```python
from build123d import *

# Parameters (mm, degrees)
F0_R     = 7
F0_R_2   = 25
F1_DEPTH = 6
F2_R     = 10


with BuildPart() as f1:
    # F0 (on Top) → F1 (new body)
    with BuildSketch(Plane.XY):
        Polygon((-28.867513, 50), (-28.867513, -50), (57.735027, 0), align=None)
        with Locations((-18, -31.176915)):
            Circle(F0_R, mode=Mode.SUBTRACT)
        Circle(F0_R_2, mode=Mode.SUBTRACT)
        with Locations((-18, 31.176915)):
            Circle(F0_R, mode=Mode.SUBTRACT)
        with Locations((36, 0)):
            Circle(F0_R, mode=Mode.SUBTRACT)
    extrude(amount=F1_DEPTH)

    # F2
    f2_edges = [f1.edges().sort_by_distance(p)[0] for p in [
        (-28.867513, -50, 3),
        (57.735027, 0, 3),
        (-28.867513, 50, 3),
    ]]
    fillet(f2_edges, radius=F2_R)


solid = f1.part
```
The listing builds one solid part. Answer for the finished solid, in the listing's coordinates (mm). Round coordinates to 2 decimals unless told otherwise and drop trailing zeros. Loops run counter-clockwise (first coordinate to the right, second up) from the corner with the lowest first, then second, coordinate; pieces in that order, holes last. Notation, with made-up numbers: (-2.5, 12) - (9.5, 12) arc R20 ccw to (9.5, 28) - close; hole circle Ø2 at (3.25, 52.25). An arc over 180 degrees is marked (long way). Return JSON: item names as keys, results as strings. Group by question number.
1. The part is cut by section C-C on y = -26. Determine the outline of the cut face in (x, z), then the cut area to 3 significant figures.
2. The part is cut by section A-A on y = 0. Determine the outline of the cut face in (x, z), then the cut area to 3 significant figures.
3. Each of these flat-tipped pins is pushed along its axis until it touches: P1, Ø1.5, axis at x = 2.5, z = 4.5, coming from the -Y side; P2, Ø1, axis at y = -33.5, z = 2.5, coming from the -X side; P3, Ø1.5, axis at x = -9, z = 3.5, coming from the -Y side. Where does it stop, or does it pass through?
4. The part is cut by section B-B on x = -23. Determine the outline of the cut face in (y, z).
5. Consider probe 1 along Y at (x, z) = (-17, 5.1); probe 2 along Y at (x, z) = (-18, 2.95); probe 3 along Y at (x, z) = (32, 5.1). Determine where each line is inside the solid, lowest interval first.
6. The part is cut by section D-D on z = 1.05. Determine the outline of the cut face in (x, y), then the cut area to 3 significant figures.
7. The mould has two halves that part along Y. Classify faces 1 (the cylindrical face through (-24.993, -30.869, 2.958)), 2 (the flat face through (-16.3, 19.2, 6)), 3 (the flat face through (14.038, -25.229, 2.958)), 4 (the cylindrical face through (47.734, 0.147, 3.042)): pulls with the +Y half, pulls with the -Y half, needs draft (parallel to the pull), parting line crosses it, or undercut.
Resolved:
{
 "1": {"outline": "(-28.87, 0) - (-22.71, 0) - (-22.71, 6) - (-28.87, 6) - close; (-13.29, 0) - (12.7, 0) - (12.7, 6) - (-13.29, 6) - close", "area": "193 mm²"},
 "2": {"outline": "(-28.87, 0) - (-25, 0) - (-25, 6) - (-28.87, 6) - close; (25, 0) - (29, 0) - (29, 6) - (25, 6) - close; (43, 0) - (47.74, 0) - (47.74, 6) - (43, 6) - close", "area": "75.6 mm²"},
 "3": {"P1": "stops at y = -32.32", "P2": "stops at x = -28.86", "P3": "stops at y = -38.96"},
 "4": {"outline": "(-41.79, 0) - (-36.08, 0) - (-36.08, 6) - (-41.79, 6) - close; (-26.28, 0) - (-9.8, 0) - (-9.8, 6) - (-26.28, 6) - close; (9.8, 0) - (26.28, 0) - (26.28, 6) - (9.8, 6) - close; (36.08, 0) - (41.79, 0) - (41.79, 6) - (36.08, 6) - close"},
 "5": {"probe 1": "y = -42.5 to -38.11, -24.25 to -18.33, 18.33 to 24.25, 38.11 to 42.5", "probe 2": "y = -42.64 to -38.18, -24.18 to -17.35, 17.35 to 24.18, 38.18 to 42.64", "probe 3": "y = -14.86 to -5.74, 5.74 to 14.86"},
 "6": {"outline": "(-28.87, -32.68) arc R10 ccw to (-13.87, -41.34) - (42.74, -8.66) arc R10 ccw to (42.74, 8.66) - (-13.87, 41.34) arc R10 ccw to (-28.87, 32.68) - close; hole circle Ø14 at (-18, -31.18); hole circle Ø50 at (0, 0); hole circle Ø14 at (-18, 31.18); hole circle Ø14 at (36, 0)", "area": "1,700 mm²"},
 "7": {"face 1": "undercut", "face 2": "needs draft", "face 3": "pulls with the -Y half", "face 4": "parting line crosses it"}
}
